Answer from the drawing. Dimensions are ordinates in mm from the lowest x, y and z of the part. Coordinates: 2 decimals unless noted, no trailing zeros. Order: outer loops, then holes, each group sorted by start corner. A loop starts at its lowest first (then second) coordinate and runs counter-clockwise, first axis right, second up. Notation, with made-up numbers: (59.25, 82.25) -> (91.25, 82.25) arc R36 ccw to (91.25, 119.25) -> close; hole circle Ø4 at (13.5, -15). An arc over 180 degrees is marked (long way). Use CSV: the item, a comma, the result in double quotes.
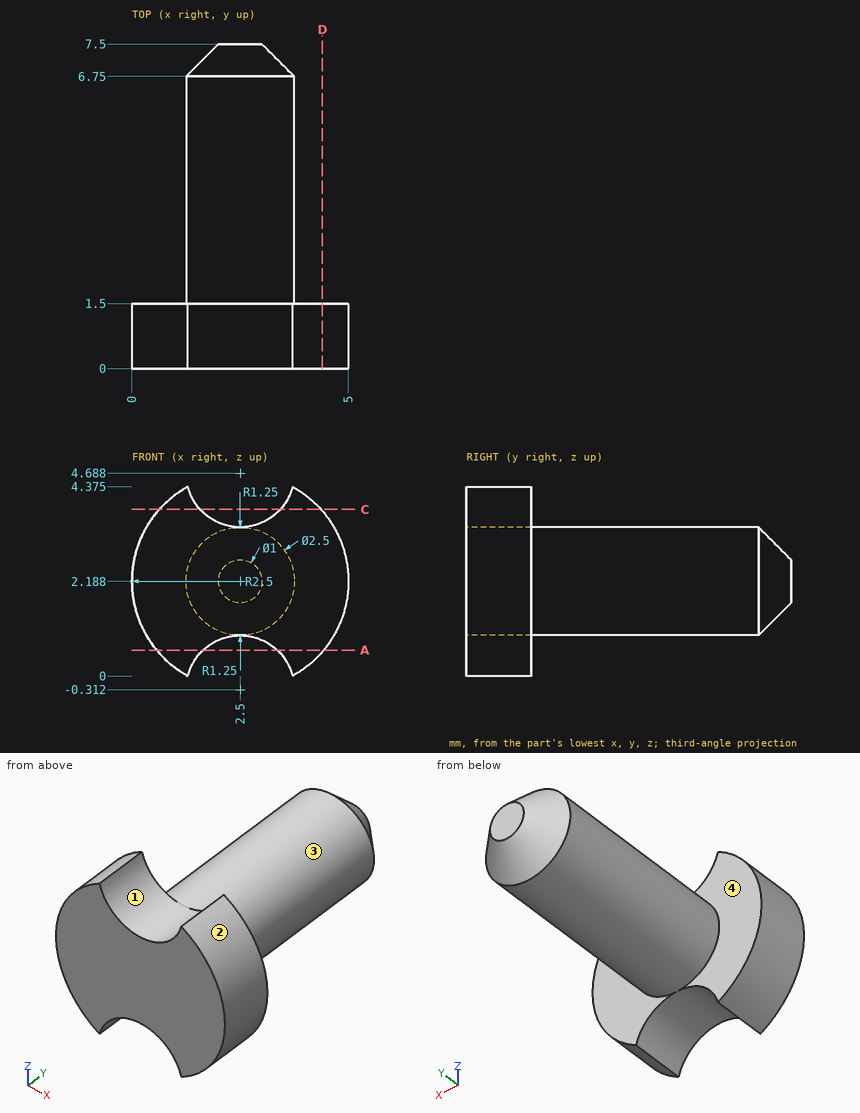
Item 1: Straight lines are drawn through the part: line 1 along Y through (x, z) = (2, 3.5); line 2 along X through (y, z) = (2.5, 2.5); line 3 along Z through (x, y) = (3.4, 4.25) (1 decimal). For each, find the intervals that lie inside material, in ascending order.
Return value:
line 1,"y = 0 to 1.5"
line 2,"x = 1.29 to 3.71"
line 3,"z = 1.3 to 3.1"
Item 2: Find section C-C, the plane z = 3.85. Give the vertices of the cut face in (x, y).
Return value:
outline,"(0.63, 0) -> (1.57, 0) -> (1.57, 1.5) -> (0.63, 1.5) -> close; (3.43, 0) -> (4.37, 0) -> (4.37, 1.5) -> (3.43, 1.5) -> close"
Item 3: Each of these flat-tipped pins is pushed along its axis until it touches: P1, Ø1.5, axis at x = 1.5, y = 4, coming from the +Z side; P2, Ø1.5, axis at x = 2.5, z = 3.5, coming from the +Y side. Where does it stop, or does it pass through?
Return value:
P1,"stops at z = 3.41"
P2,"stops at y = 7.44"
Item 4: The mould has two halves that part along X. Classify the marked faces 1, 2, 3 and 4: +X half, -X half, draft (parallel to the pull), parting line (faces both ways), or undercut.
Return value:
face 1,"undercut"
face 2,"+X half"
face 3,"parting line"
face 4,"draft"
Item 5: Find section D-D, the plane x = 4.4. Give the vertices of the cut face in (y, z).
Return value:
outline,"(0, 0.56) -> (1.5, 0.56) -> (1.5, 3.81) -> (0, 3.81) -> close"
Item 6: Find section A-A, the plane z = 0.6. Give the vertices of the cut face in (x, y) (1 decimal).
Return value:
outline,"(0.6, 0) -> (1.6, 0) -> (1.6, 1.5) -> (0.6, 1.5) -> close; (3.4, 0) -> (4.4, 0) -> (4.4, 1.5) -> (3.4, 1.5) -> close"
